For this review, take the finished solid that the model builds, in its own axes (mm). A direction names the side the tool comes from. Round coordinates to 2 decimals unless told otherwise and drop trailing zeros. Order: outer loops, then holes, each group sorted by start corner. A loop starts at its lowest first (then second) coordinate and runs counter-clockwise, first axis right, second up. Notation, with made-up numbers: (15.25, 73) -> (31.25, 73) arc R28 ccw to (31.25, 101) -> close; hole circle Ø7 at (-0.5, 27.5). An arc over 180 degrees is marked (long way). Answer in a Markdown table with one row per item.
```python
from build123d import *

# Parameters (mm, degrees)
SKETCH_1_W          = 30
SKETCH_1_H          = 30
EXTRUDE_1_DEPTH     = 3
SKETCH_2_R          = 1.75
CUT_EXTRUDE_1_DEPTH = 3
SKETCH_3_W          = 30
SKETCH_3_H          = 62.924190463
EXTRUDE_2_DEPTH     = 3
SKETCH_4_R          = 1.75
CUT_EXTRUDE_2_DEPTH = 3


with BuildPart() as part:
    # 草图1 → 凸台-拉伸1 (new body)
    with BuildSketch(Plane(origin=(0, 0, 0), x_dir=(1, 0, 0), z_dir=(0, 1, 0))):
        Rectangle(SKETCH_1_W, SKETCH_1_H)
    extrude(amount=EXTRUDE_1_DEPTH)

    # 草图2 → 切除-拉伸1 (cut)
    with BuildSketch(Plane(origin=(0, 3, 0), x_dir=(1, 0, 0), z_dir=(0, 1, 0))):
        with Locations(Location((0, -6.542683553, 0), (0, 0, 270))):
            Circle(SKETCH_2_R)
        with Locations(Location((0, 8.457316447, 0), (0, 0, 270))):
            Circle(SKETCH_2_R)
    extrude(amount=-CUT_EXTRUDE_1_DEPTH, mode=Mode.SUBTRACT)

    # 草图3 → 凸台-拉伸2 (add)
    with BuildSketch(Plane.XY.offset(15)):
        with Locations((0, 31.462095232)):
            Rectangle(SKETCH_3_W, SKETCH_3_H)
    extrude(amount=EXTRUDE_2_DEPTH)

    # 草图4 → 切除-拉伸2 (cut)
    with BuildSketch(Plane.XY.offset(18)):
        with Locations(Location((8, 43, 0), (0, 0, 180))):
            Circle(SKETCH_4_R)
        with Locations(Location((8, 18, 0), (0, 0, 180))):
            Circle(SKETCH_4_R)
        with BuildLine():
            ThreePointArc((8, 60), (10, 58), (8, 56))
            ThreePointArc((8, 56), (-1.192388155, 52.192388155), (-5, 43))
            ThreePointArc((-5, 43), (-7, 41), (-9, 43))
            ThreePointArc((-9, 43), (-4.02081528, 55.02081528), (8, 60))
        make_face()
        with BuildLine():
            ThreePointArc((-5, 18), (-7, 16), (-9, 18))
            ThreePointArc((-9, 18), (-4.02081528, 30.02081528), (8, 35))
            ThreePointArc((8, 35), (10, 33), (8, 31))
            ThreePointArc((8, 31), (-1.192388155, 27.192388155), (-5, 18))
        make_face()
    extrude(amount=-CUT_EXTRUDE_2_DEPTH, mode=Mode.SUBTRACT)


solid = part.part
```
Q1. Take a section at A-A, the plane y = 58. Write out the cut boundary in (x, z).
Answer key:
| item | result |
|---|---|
| outline | (-15, 15) -> (0, 15) -> (0, 18) -> (-15, 18) -> close; (10, 15) -> (15, 15) -> (15, 18) -> (10, 18) -> close |
Q2. Take a section at D-D, the plane x = 9. Write out the cut boundary in (y, z).
Answer key:
| item | result |
|---|---|
| outline | (0, -15) -> (3, -15) -> (3, 15) -> (16.56, 15) -> (16.56, 18) -> (0, 18) -> close; (19.44, 15) -> (31.27, 15) -> (31.27, 18) -> (19.44, 18) -> close; (34.73, 15) -> (41.56, 15) -> (41.56, 18) -> (34.73, 18) -> close; (44.44, 15) -> (56.27, 15) -> (56.27, 18) -> (44.44, 18) -> close; (59.73, 15) -> (62.92, 15) -> (62.92, 18) -> (59.73, 18) -> close |
Q3. Tool access review of faces 4 (the face through (-0.67, 1.52, -6.84)), 5 (the face through (10, 58, 17)), 6 (the face through (0, 3, 0)): name each direction out of +Z, -Z, +X, -X, +Y, -Y from which nothing blocks a thin tool from reaching the whole face with its end or side.
Answer key:
| item | result |
|---|---|
| face 4 | +Y, -Y |
| face 5 | +Z, -Z |
| face 6 | -Z, +X, -X, +Y |
Q4. To check wall thickness, follow probe 1 along Y at (x, z) = (8, 17.05); probe 2 along Y at (x, z) = (5, 8); probe 3 along Z at (x, y) = (2.25, 41). State the ranges of each line that lie inside material, in increasing order.
Answer key:
| item | result |
|---|---|
| probe 1 | y = 0 to 16.25, 19.75 to 31, 35 to 41.25, 44.75 to 56, 60 to 62.92 |
| probe 2 | y = 0 to 3 |
| probe 3 | z = 15 to 18 |
Q5. Take a section at B-B, the plane x = -7. Write out the cut boundary in (y, z), then the cut area to 3 significant figures.
Answer key:
| item | result |
|---|---|
| outline | (0, -15) -> (3, -15) -> (3, 15) -> (16, 15) -> (16, 18) -> (0, 18) -> close; (26, 15) -> (41, 15) -> (41, 18) -> (26, 18) -> close; (51, 15) -> (62.92, 15) -> (62.92, 18) -> (51, 18) -> close |
| area | 219 mm^2 |
Q6. Take a section at C-C, the plane z = 7.5. Write out the cut boundary in (x, y), then the cut area to 3 significant figures.
Answer key:
| item | result |
|---|---|
| outline | (-15, 0) -> (-1.46, 0) -> (-1.46, 3) -> (-15, 3) -> close; (1.46, 0) -> (15, 0) -> (15, 3) -> (1.46, 3) -> close |
| area | 81.2 mm^2 |
Q7. The part is to be moulded in two halves that separate along Y. For faces 1 (the face through (-4.15, 29.89, 16.52)), 2 (the face through (0.077, 1.521, 4.794)), 3 (the face through (0, 0, 1)), say which applies: +Y half, -Y half, draft (parallel to the pull), parting line (faces both ways), or undercut.
Answer key:
| item | result |
|---|---|
| face 1 | undercut |
| face 2 | draft |
| face 3 | -Y half |
Q8. Clearance check with flat-ended pins moving along their axes: pin 1 Ø12 at (x, y) = (-8.5, 25.5) entering from -Z; pin 2 Ø5.5 at (x, z) = (0, 6.54) entering from +Y. State where each tip first meets the part, or that it passes through.
Answer key:
| item | result |
|---|---|
| pin 1 | stops at z = 15 |
| pin 2 | stops at y = 3 |
